Source: CAD feature listing. Evaluate the final solid. Frame: model axes, mm. Give positions to 0.01 mm unless a question says otherwise; leave off trailing zeros. Loops run counter-clockwise (first coordinate to the right, second up) from the corner with the lowest first, then second, coordinate; pieces in that order, holes last. Notation, with made-up numbers: (-26.75, 61.25) - (23.25, 61.25) arc R25 ccw to (23.25, 93.25) - close; hole circle Ø10 at (24, 88.25). An arc over 180 degrees is marked (long way). Put each result on its own line as item: value.
```python
from build123d import *

# Parameters (mm, degrees)
BOSS_EXTRUDE1_DEPTH = 5
SKETCH2_R           = 2
SKETCH2_W           = 10
SKETCH2_H           = 80
SKETCH2_W_2         = 50
SKETCH2_H_2         = 80.000000001
CUT_EXTRUDE1_DEPTH  = 10
SKETCH4_W           = 30
SKETCH4_H           = 5.2
CUT_EXTRUDE3_DEPTH  = 10
SKETCH6_R           = 2.5
CUT_EXTRUDE5_DEPTH  = 10
SKETCH7_R           = 2
CUT_EXTRUDE6_DEPTH  = 10
CUT_EXTRUDE7_DEPTH  = 70
SKETCH10_R          = 2
CUT_EXTRUDE8_DEPTH  = 5
SKETCH11_R          = 2
CUT_EXTRUDE9_DEPTH  = 10
SKETCH16_W          = 37
SKETCH16_H          = 26
CUT_EXTRUDE10_DEPTH = 10
SKETCH17_R          = 2.15
CUT_EXTRUDE11_DEPTH = 10
SKETCH18_R          = 2
CUT_EXTRUDE12_DEPTH = 10
SKETCH24_R          = 2
CUT_EXTRUDE17_DEPTH = 5
SKETCH26_R          = 2
CUT_EXTRUDE18_DEPTH = 10


with BuildPart() as part:
    # Sketch1 → Boss-Extrude1 (new body)
    with BuildSketch(Plane.XY):
        with BuildLine():
            Line((-115, 77), (115, 77))
            ThreePointArc((115, 77), (122.071067812, 74.071067812), (125, 67))
            Line((125, 67), (125, -39))
            ThreePointArc((125, -39), (114.748737342, -63.748737342), (90, -74))
            Line((90, -74), (-90, -74))
            ThreePointArc((-90, -74), (-114.748737342, -63.748737342), (-125, -39))
            Line((-125, -39), (-125, 67))
            ThreePointArc((-125, 67), (-122.071067812, 74.071067812), (-115, 77))
        make_face()
    extrude(amount=BOSS_EXTRUDE1_DEPTH)

    # Sketch2 → Cut-Extrude1 (cut)
    with BuildSketch(Plane(origin=(0, 0, 0), x_dir=(-1, 0, 0), z_dir=(0, 0, -1))):
        with Locations((-6.6, -17.5)):
            Circle(SKETCH2_R)
        with Locations((-6.6, 17.5)):
            Circle(SKETCH2_R)
        with Locations((-40, -17.5)):
            Circle(SKETCH2_R)
        with Locations((-40, 17.5)):
            Circle(SKETCH2_R)
        with Locations((6.6, 17.5)):
            Circle(SKETCH2_R)
        with Locations((6.6, -17.5)):
            Circle(SKETCH2_R)
        with Locations((40, -17.5)):
            Circle(SKETCH2_R)
        with Locations((40, 17.5)):
            Circle(SKETCH2_R)
        with Locations((-120, 0)):
            Rectangle(SKETCH2_W, SKETCH2_H)
        with Locations((-70, -1e-09)):
            Rectangle(SKETCH2_W_2, SKETCH2_H_2)
        with Locations((120, 0)):
            Rectangle(SKETCH2_W, SKETCH2_H)
        with Locations((70, -1e-09)):
            Rectangle(SKETCH2_W_2, SKETCH2_H_2)
    extrude(amount=-CUT_EXTRUDE1_DEPTH, mode=Mode.SUBTRACT)

    # Sketch4 → Cut-Extrude3 (cut)
    with BuildSketch(Plane(origin=(0, 0, 0), x_dir=(-1, 0, 0), z_dir=(0, 0, -1))):
        with Locations((0, 37.6)):
            Rectangle(SKETCH4_W, SKETCH4_H)
        with Locations((0, -37.6)):
            Rectangle(SKETCH4_W, SKETCH4_H)
    extrude(amount=-CUT_EXTRUDE3_DEPTH, mode=Mode.SUBTRACT)

    # Sketch6 → Cut-Extrude5 (cut)
    with BuildSketch(Plane(origin=(0, 0, 0), x_dir=(-1, 0, 0), z_dir=(0, 0, -1))):
        with Locations((-102.2, -25.5)):
            Circle(SKETCH6_R)
        with Locations((-102.2, 25.5)):
            Circle(SKETCH6_R)
        with Locations((102.2, -25.5)):
            Circle(SKETCH6_R)
        with Locations((102.2, 25.5)):
            Circle(SKETCH6_R)
    extrude(amount=-CUT_EXTRUDE5_DEPTH, mode=Mode.SUBTRACT)

    # Sketch7 → Cut-Extrude6 (cut)
    with BuildSketch(Plane(origin=(0, 0, 0), x_dir=(-1, 0, 0), z_dir=(0, 0, -1))):
        with Locations((29.9, 37.5)):
            Circle(SKETCH7_R)
        with Locations((-29.9, -37.5)):
            Circle(SKETCH7_R)
        with Locations((-29.9, 37.5)):
            Circle(SKETCH7_R)
        with Locations((29.9, -37.5)):
            Circle(SKETCH7_R)
    extrude(amount=-CUT_EXTRUDE6_DEPTH, mode=Mode.SUBTRACT)

    # Sketch8 → Cut-Extrude7 (cut)
    with BuildSketch(Plane(origin=(0, 0, 0), x_dir=(-1, 0, 0), z_dir=(0, 0, -1))):
        with BuildLine():
            Line((5.5, 71), (-5.5, 71))
            ThreePointArc((-5.5, 71), (-7.621320344, 70.121320344), (-8.5, 68))
            Line((-8.5, 68), (-8.5, 53))
            ThreePointArc((-8.5, 53), (-7.621320344, 50.878679656), (-5.5, 50))
            Line((-5.5, 50), (5.5, 50))
            ThreePointArc((5.5, 50), (7.621320344, 50.878679656), (8.5, 53))
            Line((8.5, 53), (8.5, 68))
            ThreePointArc((8.5, 68), (7.621320344, 70.121320344), (5.5, 71))
        make_face()
    extrude(amount=-CUT_EXTRUDE7_DEPTH, mode=Mode.SUBTRACT)

    # Sketch10 → Cut-Extrude8 (cut)
    with BuildSketch(Plane(origin=(0, 0, 0), x_dir=(-1, 0, 0), z_dir=(0, 0, -1))):
        with Locations((13, 60.5)):
            Circle(SKETCH10_R)
        with Locations((-13, 60.5)):
            Circle(SKETCH10_R)
    extrude(amount=-CUT_EXTRUDE8_DEPTH, mode=Mode.SUBTRACT)

    # Sketch11 → Cut-Extrude9 (cut)
    with BuildSketch(Plane(origin=(0, 0, 0), x_dir=(-1, 0, 0), z_dir=(0, 0, -1))):
        with Locations((-17, -62.5)):
            Circle(SKETCH11_R)
        with Locations((17, -62.5)):
            Circle(SKETCH11_R)
        with BuildLine():
            Line((-9, -54), (9, -54))
            ThreePointArc((9, -54), (11.121320344, -54.878679656), (12, -57))
            Line((12, -57), (12, -68))
            ThreePointArc((12, -68), (11.121320344, -70.121320344), (9, -71))
            Line((9, -71), (-9, -71))
            ThreePointArc((-9, -71), (-11.121320344, -70.121320344), (-12, -68))
            Line((-12, -68), (-12, -57))
            ThreePointArc((-12, -57), (-11.121320344, -54.878679656), (-9, -54))
        make_face()
    extrude(amount=-CUT_EXTRUDE9_DEPTH, mode=Mode.SUBTRACT)

    # Sketch16 → Cut-Extrude10 (cut)
    with BuildSketch(Plane(origin=(0, 0, 0), x_dir=(-1, 0, 0), z_dir=(0, 0, -1))):
        with Locations((-91.5, 64)):
            Rectangle(SKETCH16_W, SKETCH16_H)
        with Locations((91.5, 64)):
            Rectangle(SKETCH16_W, SKETCH16_H)
    extrude(amount=-CUT_EXTRUDE10_DEPTH, mode=Mode.SUBTRACT)

    # Sketch17 → Cut-Extrude11 (cut)
    with BuildSketch(Plane(origin=(0, 0, 0), x_dir=(-1, 0, 0), z_dir=(0, 0, -1))):
        with Locations((67.6, 65.6)):
            Circle(SKETCH17_R)
        with Locations((67.6, 55.4)):
            Circle(SKETCH17_R)
        with Locations((115.4, 55.4)):
            Circle(SKETCH17_R)
        with Locations((115.4, 65.6)):
            Circle(SKETCH17_R)
        with Locations((-115.4, 65.6)):
            Circle(SKETCH17_R)
        with Locations((-115.4, 55.4)):
            Circle(SKETCH17_R)
        with Locations((-67.6, 55.4)):
            Circle(SKETCH17_R)
        with Locations((-67.6, 65.6)):
            Circle(SKETCH17_R)
    extrude(amount=-CUT_EXTRUDE11_DEPTH, mode=Mode.SUBTRACT)

    # Sketch18 → Cut-Extrude12 (cut)
    with BuildSketch(Plane(origin=(0, 0, 0), x_dir=(-1, 0, 0), z_dir=(0, 0, -1))):
        with Locations((-43.2, 68.5)):
            Circle(SKETCH18_R)
        with Locations((43.2, 68.5)):
            Circle(SKETCH18_R)
    extrude(amount=-CUT_EXTRUDE12_DEPTH, mode=Mode.SUBTRACT)

    # Sketch24 → Cut-Extrude17 (cut)
    with BuildSketch(Plane(origin=(0, 0, 0), x_dir=(-1, 0, 0), z_dir=(0, 0, -1))):
        with Locations((-42.8, -52.5)):
            Circle(SKETCH24_R)
        with Locations((42.8, -52.5)):
            Circle(SKETCH24_R)
    extrude(amount=-CUT_EXTRUDE17_DEPTH, mode=Mode.SUBTRACT)

    # Sketch26 → Cut-Extrude18 (cut)
    with BuildSketch(Plane(origin=(0, 0, 0), x_dir=(-1, 0, 0), z_dir=(0, 0, -1))):
        with Locations((-112, -51)):
            Circle(SKETCH26_R)
        with Locations((-65, -51)):
            Circle(SKETCH26_R)
        with Locations((65, -51)):
            Circle(SKETCH26_R)
        with Locations((112, -51)):
            Circle(SKETCH26_R)
    extrude(amount=-CUT_EXTRUDE18_DEPTH, mode=Mode.SUBTRACT)


solid = part.part
```
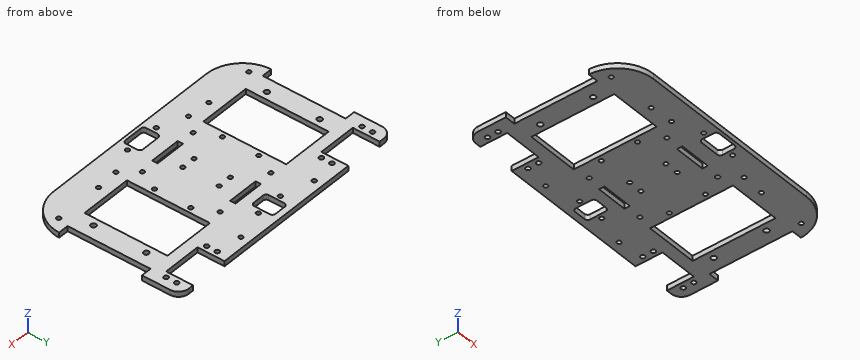
1) Section query B-B, the plane x = 51.5. Output: boundary loops of the cut face in (y, z).
Check result:
outline: (-74, 0) - (-40, 0) - (-40, 5) - (-74, 5) - close; (40, 0) - (77, 0) - (77, 5) - (40, 5) - close
2) Section query A-A, the plane y = 25.5. Output: boundary loops of the cut face in (x, z).
Check result:
outline: (-115, 0) - (-104.7, 0) - (-104.7, 5) - (-115, 5) - close; (-99.7, 0) - (-95, 0) - (-95, 5) - (-99.7, 5) - close; (-45, 0) - (45, 0) - (45, 5) - (-45, 5) - close; (95, 0) - (99.7, 0) - (99.7, 5) - (95, 5) - close; (104.7, 0) - (115, 0) - (115, 5) - (104.7, 5) - close
3) Material intervals for line 1 along Y through (x, z) = (-0.5, 3.9); line 2 along Y through (x, z) = (29.9, 3); line 3 along X through (y, z) = (25, 2.45), sorted ascending. Write a range as [from, to].
Check result:
line 1: [-74, -71], [-54, -40.2], [-35, 35], [40.2, 50], [71, 77]
line 2: [-74, -39.5], [-35.5, 35.5], [39.5, 77]
line 3: [-115, -104.65], [-99.75, -95], [-45, 45], [95, 99.75], [104.65, 115]
4) Pin query (flat end, axial travel): P1, Ø2.5, axis at x = 86, z = 2.5, coming from the +Y side; P2, Ø2.5, axis at y = -15.5, z = 2, coming from the -X side. Return the tip coordinate at first contact, or that it passes through.
Check result:
P1: y = 51
P2: x = -115
5) Section query C-C, the plane x = 102.2. Output: boundary loops of the cut face in (y, z), plus the area to 3 significant figures.
Check result:
outline: (-71.8, 0) - (-28, 0) - (-28, 5) - (-71.8, 5) - close; (-23, 0) - (23, 0) - (23, 5) - (-23, 5) - close; (28, 0) - (51, 0) - (51, 5) - (28, 5) - close
area: 564 mm²
6) Section query D-D, the plane z = 2.7. State how many separate pieces and enclosed holes the cut face has, plus the area to 3 significant figures.
Check result:
separate pieces: 1
enclosed holes: 42
area: 24,100 mm²
